Verification items for the finished model (mm, model axes). A direction names the side the tool comes from. Round coordinates to 2 decimals unless told otherwise and drop trailing zeros. Loops run counter-clockwise (first coordinate to the right, second up) from the corner with the lowest first, then second, coordinate; pieces in that order, holes last. Notation, with made-up numbers: (30.5, -18) -> (85.5, -18) arc R30 cw to (85.5, 19) -> close; hole circle Ø7 at (-39.5, -15.5). An arc over 180 degrees is marked (long way). Write item = value, one per line. Start each with the question number.
```python
from build123d import *

# Parameters (mm, degrees)
F0_W     = 30
F0_H     = 30
F1_DEPTH = 10
F2_SIZE  = 0.29999


# Not quite as in the source:
# - a fillet or chamfer is up to 0.001 mm smaller than in the source, because OpenCascade refuses the exact size


with BuildPart() as f1:
    # F0 (on Top) → F1 (new body)
    with BuildSketch(Plane.XY):
        with Locations((8.7794362941, 10.8101805312)):
            Rectangle(F0_W, F0_H)
        with BuildLine():
            Line((13.2, 20), (19.5, 20))
            ThreePointArc((19.5, 20), (19.8535533906, 19.8535533906), (20, 19.5))
            Line((20, 19.5), (20, 13.2))
            Line((20, 13.2), (18.6, 13.2))
            Line((18.6, 13.2), (18.6, 16.8857864376))
            ThreePointArc((18.6, 16.8857864376), (18.4148050297, 17.1629502974), (18.0878679656, 17.097918472))
            Line((18.0878679656, 17.097918472), (14.0849274668, 13.0949779732))
            ThreePointArc((14.0849274668, 13.0949779732), (13.8016579584, 12.5262720767), (13.918171677, 11.9016981704))
            ThreePointArc((13.918171677, 11.9016981704), (14.4115666356, 10), (13.918171677, 8.0983018296))
            ThreePointArc((13.918171677, 8.0983018296), (13.8016579584, 7.4737279233), (14.0849274668, 6.9050220268))
            Line((14.0849274668, 6.9050220268), (17.9171572875, 3.0727922061))
            ThreePointArc((17.9171572875, 3.0727922061), (18.3530733729, 2.9860831056), (18.6, 3.3556349186))
            Line((18.6, 3.3556349186), (18.6, 6.8))
            Line((18.6, 6.8), (20, 6.8))
            Line((20, 6.8), (20, 0.5))
            ThreePointArc((20, 0.5), (19.8535533906, 0.1464466094), (19.5, 0))
            Line((19.5, 0), (13.2, 0))
            Line((13.2, 0), (13.2, 1.4))
            Line((13.2, 1.4), (16.6443650814, 1.4))
            ThreePointArc((16.6443650814, 1.4), (17.0139168944, 1.6469266271), (16.9272077939, 2.0828427125))
            Line((16.9272077939, 2.0828427125), (13.0949779732, 5.9150725332))
            ThreePointArc((13.0949779732, 5.9150725332), (12.5262720767, 6.1983420416), (11.9016981704, 6.081828323))
            ThreePointArc((11.9016981704, 6.081828323), (10, 5.5884333644), (8.0983018296, 6.081828323))
            ThreePointArc((8.0983018296, 6.081828323), (7.4737279233, 6.1983420416), (6.9050220268, 5.9150725332))
            Line((6.9050220268, 5.9150725332), (3.0727922061, 2.0828427125))
            ThreePointArc((3.0727922061, 2.0828427125), (2.9860831056, 1.6469266271), (3.3556349186, 1.4))
            Line((3.3556349186, 1.4), (6.8, 1.4))
            Line((6.8, 1.4), (6.8, 0))
            Line((6.8, 0), (0.5, 0))
            ThreePointArc((0.5, 0), (0.1464466094, 0.1464466094), (0, 0.5))
            Line((0, 0.5), (0, 6.8))
            Line((0, 6.8), (1.4, 6.8))
            Line((1.4, 6.8), (1.4, 3.3556349186))
            ThreePointArc((1.4, 3.3556349186), (1.6469266271, 2.9860831056), (2.0828427125, 3.0727922061))
            Line((2.0828427125, 3.0727922061), (5.9150725332, 6.9050220268))
            ThreePointArc((5.9150725332, 6.9050220268), (6.1983420416, 7.4737279233), (6.081828323, 8.0983018296))
            ThreePointArc((6.081828323, 8.0983018296), (5.5884333644, 10), (6.081828323, 11.9016981704))
            ThreePointArc((6.081828323, 11.9016981704), (6.1983420416, 12.5262720767), (5.9150725332, 13.0949779732))
            Line((5.9150725332, 13.0949779732), (2.0828427125, 16.9272077939))
            ThreePointArc((2.0828427125, 16.9272077939), (1.6469266271, 17.0139168944), (1.4, 16.6443650814))
            Line((1.4, 16.6443650814), (1.4, 13.2))
            Line((1.4, 13.2), (0, 13.2))
            Line((0, 13.2), (0, 19.5))
            ThreePointArc((0, 19.5), (0.1464466094, 19.8535533906), (0.5, 20))
            Line((0.5, 20), (6.8, 20))
            Line((6.8, 20), (6.8, 18.6))
            Line((6.8, 18.6), (3.3556349186, 18.6))
            ThreePointArc((3.3556349186, 18.6), (2.9860831056, 18.3530733729), (3.0727922061, 17.9171572875))
            Line((3.0727922061, 17.9171572875), (6.9050220268, 14.0849274668))
            ThreePointArc((6.9050220268, 14.0849274668), (7.4737279233, 13.8016579584), (8.0983018296, 13.918171677))
            ThreePointArc((8.0983018296, 13.918171677), (10, 14.4115666356), (11.9016981704, 13.918171677))
            ThreePointArc((11.9016981704, 13.918171677), (12.5262720767, 13.8016579584), (13.0949779732, 14.0849274668))
            Line((13.0949779732, 14.0849274668), (17.097918472, 18.0878679656))
            ThreePointArc((17.097918472, 18.0878679656), (17.1629502974, 18.4148050297), (16.8857864376, 18.6))
            Line((16.8857864376, 18.6), (13.2, 18.6))
            Line((13.2, 18.6), (13.2, 20))
        make_face(mode=Mode.SUBTRACT)
    extrude(amount=F1_DEPTH)

    # F2 (size 0.3 in the source; OpenCascade refuses exactly that, so slightly less here)
    f2_edges = [f1.edges().sort_by_distance(p)[0] for p in [
        (0, 16.35, 10),
        (4.988907, 16.001042, 10),
        (3.998958, 15.011093, 10),
        (7.473728, 6.198342, 10),
        (14.411567, 10, 10),
        (19.3, 13.2, 10),
        (16.35, 20, 10),
        (13.2, 19.3, 10),
        (6.8, 19.3, 10),
        (20, 3.65, 10),
        (13.2, 0.7, 10),
        (6.8, 0.7, 10),
        (0.7, 6.8, 10),
        (19.3, 6.8, 10),
        (0, 3.65, 10),
    ]]
    chamfer(f2_edges, length=F2_SIZE)


solid = f1.part
```
(1) Draft check along X on faces 4 (the flat face through (9, 25.81, 5)), 5 (the flat face through (-6.221, 11, 5)), 6 (the cylindrical face through (6.2, 7.5, 4.8)). Enter one of: +X half, -X half, draft (parallel to the pull), parting line (faces both ways), or undercut.
(2) Section check A-A on x = 1. Enter the section's corners in (y, z).
(3) Scan lines: line 1 (X direction, y = 0.5, z = 2.75); line 2 (Y direction, x = 19, z = 7.25); line 3 (X direction, y = 13.25, z = 5.5). Record each from-to range of solid material in increasing order. Write a range as [from, to].
(4) Access from +Z, -Z, +X, -X, +Y, -Y to the whole of each face (thin tool, end or side, straight path). Record for faces 1 (the flat face through (23.779, 11, 5)), 2 (the flat face through (14.961, 16.166, 9.852)), 3 (the flat face through (15.07, 16.06, 4.78)).
Computed values:
q1.face_4 = draft
q1.face_5 = -X half
q1.face_6 = undercut
q2.outline = (-4.19, 0) -> (0, 0) -> (0, 9.7) -> (-0.3, 10) -> (-4.19, 10) -> close; (6.8, 0) -> (13.2, 0) -> (13.2, 10) -> (7.1, 10) -> (6.8, 9.7) -> close; (20, 0) -> (25.81, 0) -> (25.81, 10) -> (20.3, 10) -> (20, 9.7) -> close
q3.line_1 = [-6.22, 0], [6.8, 13.2], [20, 23.78]
q3.line_2 = [-4.19, 0], [6.8, 13.2], [20, 25.81]
q3.line_3 = [-6.22, 0], [1.4, 5.76], [14.24, 18.6], [20, 23.78]
q4.face_1 = +Z, -Z, +X, +Y, -Y
q4.face_2 = +Z
q4.face_3 = +Z, -Z
